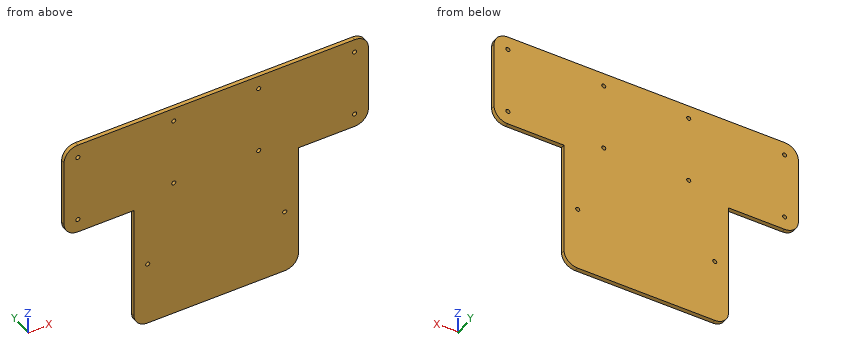
```python
from build123d import *

# Parameters (mm, degrees)
SKETCH1_R           = 1.5
BOSS_EXTRUDE1_DEPTH = 3
FILLET1_R           = 10


with BuildPart() as part:
    # Sketch1 → Boss-Extrude1 (new body)
    with BuildSketch(Plane(origin=(0, 0, 0), x_dir=(1, 0, 0), z_dir=(0, 1, 0))):
        Polygon((-60, 130), (60, 130), (60, 35), (111, 35), (111, -35), (-111, -35), (-111, 35), (-60, 35), align=None)
        with Locations(Location((-50, 82.5, 0), (0, 0, 270))):
            Circle(SKETCH1_R, mode=Mode.SUBTRACT)
        with Locations(Location((-101, 25, 0), (0, 0, 270))):
            Circle(SKETCH1_R, mode=Mode.SUBTRACT)
        with Locations(Location((-101, -25, 0), (0, 0, 90))):
            Circle(SKETCH1_R, mode=Mode.SUBTRACT)
        with Locations(Location((-31, 25, 0), (0, 0, 270))):
            Circle(SKETCH1_R, mode=Mode.SUBTRACT)
        with Locations(Location((-31, -25, 0), (0, 0, 90))):
            Circle(SKETCH1_R, mode=Mode.SUBTRACT)
        with Locations(Location((101, 25, 0), (0, 0, 90))):
            Circle(SKETCH1_R, mode=Mode.SUBTRACT)
        with Locations(Location((101, -25, 0), (0, 0, 270))):
            Circle(SKETCH1_R, mode=Mode.SUBTRACT)
        with Locations(Location((31, -25, 0), (0, 0, 270))):
            Circle(SKETCH1_R, mode=Mode.SUBTRACT)
        with Locations(Location((31, 25, 0), (0, 0, 90))):
            Circle(SKETCH1_R, mode=Mode.SUBTRACT)
        with Locations(Location((50, 82.5, 0), (0, 0, 90))):
            Circle(SKETCH1_R, mode=Mode.SUBTRACT)
    extrude(amount=BOSS_EXTRUDE1_DEPTH)

    # Fillet1
    fillet1_edges = [part.edges().sort_by_distance(p)[0] for p in [
        (111, 1.5, -35),
        (111, 1.5, 35),
        (-111, 1.5, 35),
        (-111, 1.5, -35),
        (-60, 1.5, -130),
        (60, 1.5, -130),
    ]]
    fillet(fillet1_edges, radius=FILLET1_R)


solid = part.part
```
Input: part model. Units: mm. Frame: model coordinates. Coordinates: 2 decimals unless noted, no trailing zeros. Write each loop counter-clockwise with the first axis right and the second up, starting at its lowest first coordinate (ties: lowest second). Pieces come first, ordered by that corner, then holes. Notation, with made-up numbers: (16.5, 84.5) -> (21.5, 84.5) arc R23 cw to (21.5, 123.5) -> close; hole circle Ø7 at (-22, 88.5). An arc over 180 degrees is marked (long way). Answer as a JSON object with one key per item and string values.
1. First-contact query: P1, Ø2.5, axis at x = 31, z = -25, coming from the +Y side; P2, Ø1.5, axis at y = 2, z = -59.5, coming from the +X side; P3, Ø1, axis at y = 0.5, z = -105.5, coming from the -X side. Flat tips, straight axial feed; report the tip coordinate or a pass-through.
Result set:
{"P1": "passes through", "P2": "stops at x = 60", "P3": "stops at x = -60"}
2. Section C-C on z = -51. Return the cut outline in (x, y), then the cut area to 3 significant figures.
Result set:
{"outline": "(-60, 0) -> (60, 0) -> (60, 3) -> (-60, 3) -> close", "area": "360 mm2"}
3. Section A-A on y = 0.6. Count the separate pieces of the cut face and the enclosed holes in it, then the cut area to 3 significant figures.
Result set:
{"separate pieces": "1", "enclosed holes": "10", "area": "26,700 mm2"}
4. Section B-B on x = -84.5. Return the cut outline in (y, z), then the cut area to 3 significant figures.
Result set:
{"outline": "(0, -35) -> (3, -35) -> (3, 35) -> (0, 35) -> close", "area": "210 mm2"}
5. Material intervals for line 1 (X direction, y = 0.9, z = 25); line 2 (X direction, y = 1.3, z = -82.5); line 3 (Z direction, x = 100, y = 1.1), sorted ascending. Write a range as from..to.
Result set:
{"line 1": "x = -111..-102.5, -99.5..-32.5, -29.5..29.5, 32.5..99.5, 102.5..111", "line 2": "x = -60..-51.5, -48.5..48.5, 51.5..60", "line 3": "z = -35..-26.12, -23.88..23.88, 26.12..35"}
